Geometry check sheet. Reference: the model listing, model coordinates, mm. Give positions to 0.01 mm unless a question says otherwise; leave off trailing zeros. Write each loop counter-clockwise with the first axis right and the second up, starting at its lowest first coordinate (ties: lowest second). Pieces come first, ordered by that corner, then holes. Notation, with made-up numbers: (-36.75, -15.5) -> (-15.75, -15.5) arc R32 ccw to (-15.75, 14.5) -> close; hole circle Ø10 at (-7, 82). An arc over 180 degrees is marked (long way). Use a Markdown table: item, result. Add a question column.
Autodesk Inventor part; units mm, degrees
ref_plane "YZ Plane" through (0, 0, 0) normal (1, 0, 0) x (0, 1, 0)
ref_plane "XZ Plane" through (0, 0, 0) normal (0, 1, 0) x (-1, 0, 0)
ref_plane "XY Plane" through (0, 0, 0) normal (0, 0, 1) x (1, 0, 0)
sketch "Sketch1" plane through (0, 0, 0) normal (0, 1, 0) x (-1, 0, 0)
  line L0 (0, 0) -> (8, 0)
  line L1 (8, -10) -> (0, -10)
  line L2 (0, -10) -> (0, 0)
  line L3 (8, -1) -> (1, -1)
  line L4 (1, -1) -> (1, -9)
  line L5 (1, -9) -> (8, -9)
  line L6 (8, 0) -> (8, -1)
  line L7 (8, -9) -> (8, -10)
  dimension "d0" = 1
  dimension "d1" = 1
  dimension "d2" = 1
  dimension "d3" = 10
  dimension "d4" = 8
extrude "Extrusion1" add sketch "Sketch1" along normal blind 339
sketch "Sketch2" plane through (0, 0, 0) normal (1, 0, 0) x (0, 0, -1)
  line L0 (0, 0) -> (10, 0)
  line L1 (0, 0) -> (0, 339)
  point P0 (5, 9)
  dimension "d7" = 9
  dimension "d8" = 5
hole "Hole1" at (0, 9, -5) direction (-1, 0, 0) diameter 3 depth 8 tip angle 118
sketch "Sketch3" plane through (0, 0, 0) normal (1, 0, 0) x (0, 0, -1)
  line L0 (0, 0) -> (0, 339)
  line L1 (0, 339) -> (10, 339)
  point P0 (5, 206.5)
  point P1 (5, 339)
  dimension "d16" = 5
  dimension "d17" = 132.5
hole "Hole2" [suppressed]
sketch "Sketch5" plane through (0, 0, 0) normal (1, 0, 0) x (0, 0, -1)
  line L0 (0, 0) -> (0, 339)
  circle A0 centre (5, 9) radius 1.5
  point P0 (5, 151)
  dimension "d25" = 5
  dimension "d26" = 142
hole "Hole3" at (0, 151, -5) direction (-1, 0, 0) diameter 3 depth 8 tip angle 118
sketch "Sketch11" plane through (0, 0, 0) normal (0, -1, 0) x (1, 0, 0)
  circle A0 centre (-6.5, -5) radius 1.5
  line L0 (-8, -10) -> (-8, -9)
  line L1 (0, -10) -> (-8, -10)
  line L2 (-8, -9) -> (-1, -9)
  line L3 (-1, -9) -> (-9.5, -9)
  line L4 (-9.5, -9) -> (-9.5, -1)
  line L5 (-9.5, -1) -> (-1, -1)
  line L6 (-1, -1) -> (-1, -9)
  point P0 (0, 0)
  point P1 (-8, -9.5)
  dimension "d63" = 3
  dimension "d64" = 1.5
  dimension "d65" = 5
  dimension "d66" = 3
extrude "Extrusion3" add sketch "Sketch11" against normal blind 1
properties part number "Stringer" material "Aluminum"
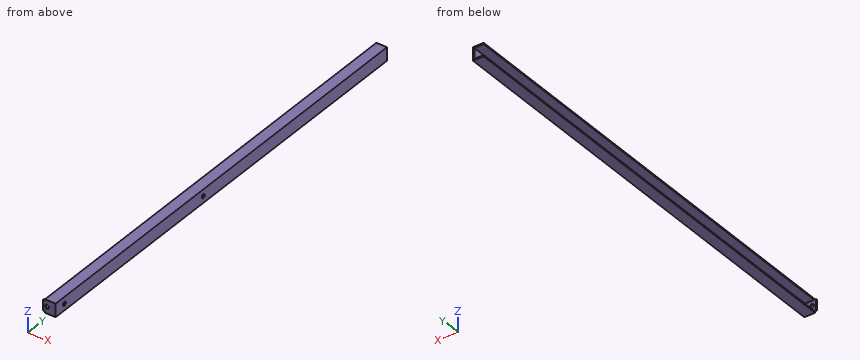
1) Sectioned sample at A-A, the plane z = -5. Enter the section's corners in (x, y).
2) Gauge pin test, flat ends, axial feed: P1, Ø1.1, axis at y = 249, z = -0.5, coming from the -X side; P2, Ø0.8, axis at x = -8.5, y = 0.5, coming from the +Z side; P3, Ø1.5, axis at x = -8.5, z = -5.5, coming from the +Y side. Record the tip position at first contact, or that the pin passes through.
3) Sectioned sample at B-B, the plane x = -6.5. Enter the section's corners in (y, z), and give its area (3 significant figures).
4) Sectioned sample at C-C, the plane y = 253. Enter the section's corners in (x, z).
5) Material ranges on probe 1 along Y at (x, z) = (-0.5, -5); probe 2 along Z at (x, y) = (-1.75, 272); probe 3 along Z at (x, y) = (-0.3, 9), recorded low to high. Write a range as [from, to].
Check values:
| question | item | result |
|---|---|---|
| 1 | outline | (-9.5, 0) -> (-8, 0) -> (-8, 1) -> (-9.5, 1) -> close; (-5, 0) -> (0, 0) -> (0, 7.5) -> (-1, 7.5) -> (-1, 1) -> (-5, 1) -> close; (-1, 10.5) -> (0, 10.5) -> (0, 149.5) -> (-1, 149.5) -> close; (-1, 152.5) -> (0, 152.5) -> (0, 339) -> (-1, 339) -> close |
| 2 | P1 | x = -8 |
| 2 | P2 | z = -1 |
| 2 | P3 | y = 1 |
| 3 | outline | (0, -10) -> (339, -10) -> (339, -9) -> (1, -9) -> (1, -6.5) -> (0, -6.5) -> close; (0, -3.5) -> (1, -3.5) -> (1, -1) -> (339, -1) -> (339, 0) -> (0, 0) -> close |
| 3 | area | 683 mm² |
| 4 | outline | (-8, -10) -> (0, -10) -> (0, 0) -> (-8, 0) -> (-8, -1) -> (-1, -1) -> (-1, -9) -> (-8, -9) -> close |
| 5 | probe 1 | [0, 7.5], [10.5, 149.5], [152.5, 339] |
| 5 | probe 2 | [-10, -9], [-1, 0] |
| 5 | probe 3 | [-10, -6.5], [-3.5, 0] |
